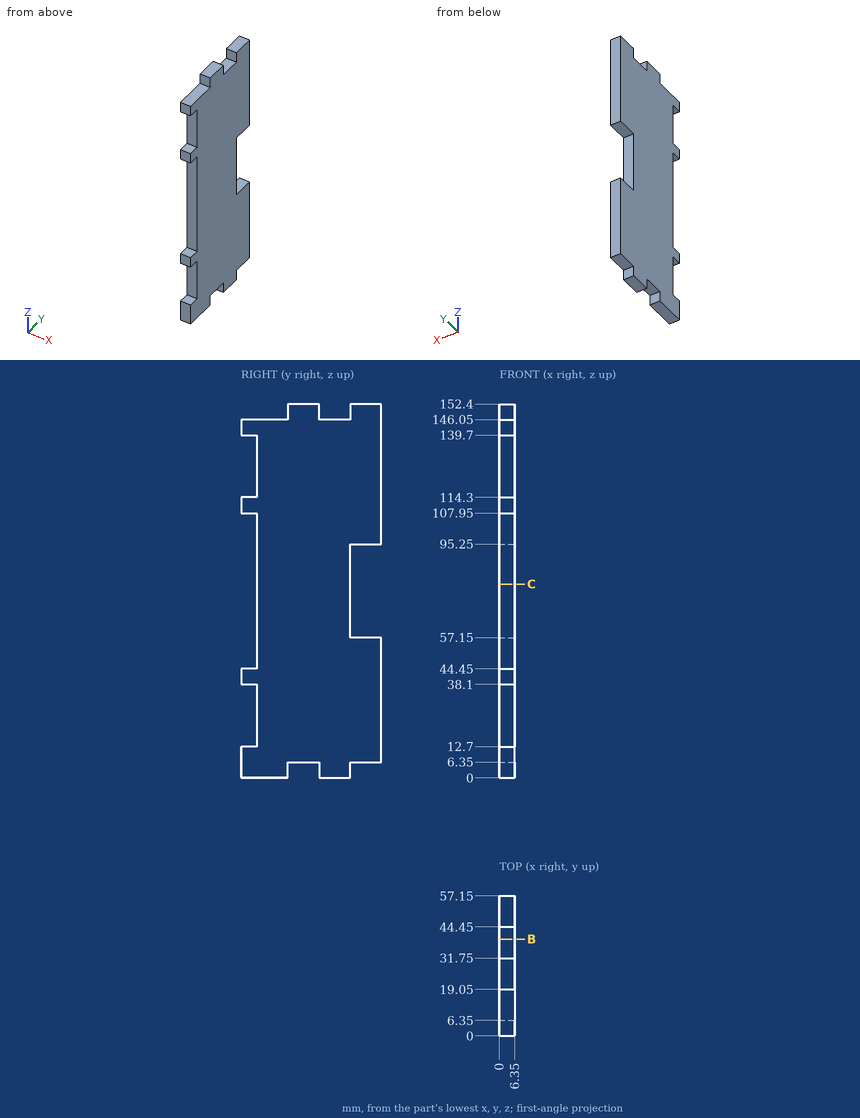
Input: dimensioned drawing with shaded views. Units: mm. Origin: part minimum x, y, z. Round coordinates to 2 decimals unless told otherwise and drop trailing zeros. Order: outer loops, then holes, each group sorted by start corner. A loop starts at its lowest first (then second) coordinate and runs counter-clockwise, first axis right, second up. Notation, with made-up numbers: (58.5, -34) -> (105.5, -34) arc R21 cw to (105.5, -8) -> close; hole circle Ø2 at (89, -24.75). An arc over 180 degrees is marked (long way). Put each result on its own line as item: value. Start each with the question number.
Q1. Section B-B on y = 39.5. Return the cut outline in (x, z).
Q2. Section C-C on z = 79. Return the cut outline in (x, y).
Q3. First-contact query: pin 1 (1.9 mm diameter, centred on x = 4, y = 1.5, fed in from -Z); pin 2 (3 mm diameter, centred on x = 3.5, z = 78.5, fed in from +Y); pin 3 (3 mm diameter, centred on x = 3.5, z = 22.5, fed in from -Y); pin 4 (1.9 mm diameter, centred on x = 3.5, z = 150, fed in from -Y). Flat tips, straight axial feed; report the tip coordinate or a pass-through.
Q4. Line query: probe 1 along Z at (x, y) = (5.5, 51.5); probe 2 along Y at (x, z) = (1, 79); probe 3 along Z at (x, y) = (1.25, 38). Output: solid intervals per line, ascending.
Ans:
1. outline: (0, 0) -> (6.35, 0) -> (6.35, 146.05) -> (0, 146.05) -> close
2. outline: (0, 6.35) -> (6.35, 6.35) -> (6.35, 44.45) -> (0, 44.45) -> close
3. pin 1: stops at z = 0
3. pin 2: stops at y = 44.45
3. pin 3: stops at y = 6.35
3. pin 4: stops at y = 19.05
4. probe 1: z = 6.35 to 57.15, 95.25 to 152.4
4. probe 2: y = 6.35 to 44.45
4. probe 3: z = 0 to 146.05
